CAD build for the part. Positions are in the model's coordinates, mm. A direction names the side the tool comes from. Coordinates: 2 decimals unless noted, no trailing zeros. Order: outer loops, then holes, each group sorted by start corner. A loop starts at its lowest first (then second) coordinate and runs counter-clockwise, first axis right, second up. Notation, with made-up numbers: (76, 47) - (87, 47) arc R14 cw to (87, 56) - close; hole circle Ø9 at (15.5, 49.25). An arc over 180 degrees is marked (long way). Return JSON: item names as keys, results as strings.
Autodesk Inventor part; units mm, degrees
ref_plane "YZ Plane" through (0, 0, 0) normal (1, 0, 0) x (0, 1, 0)
ref_plane "XZ Plane" through (0, 0, 0) normal (0, 1, 0) x (-1, 0, 0)
ref_plane "XY Plane" through (0, 0, 0) normal (0, 0, 1) x (1, 0, 0)
sketch "Sketch2" plane through (0, 0, 0) normal (1, 0, 0) x (0, 1, 0)
  line L0 (16.0342, 2.2983) -> (13.213, 1.278)
  line L1 (13.213, 1.278) -> (17.9745, -11.8874)
  line L2 (17.9745, -11.8874) -> (20.7956, -10.8671)
  line L3 (20.7956, -10.8671) -> (16.0342, 2.2983)
  line L4 (16.8006, 6.0599) -> (24.0368, -13.9485)
  line L5 (14.6738, 6.0599) -> (16.8006, 6.0599)
  line L6 (24.0368, -13.9485) -> (19.3349, -15.649)
  line L7 (19.3349, -15.649) -> (14.6738, -15.649)
  line L8 (22.156, -14.6287) -> (14.6738, 6.0599) construction
  line L9 (17.9745, -11.8874) -> (11.3917, -14.2681) construction
  line L10 (11.3917, -14.2681) -> (6.6303, -1.1027) construction
  line L11 (6.6303, -1.1027) -> (13.213, 1.278) construction
  line L12 (6.6738, 6.0599) -> (3.6738, 6.0599)
  line L13 (3.6738, 6.0599) -> (3.6738, -15.649)
  line L14 (3.6738, -15.649) -> (6.6738, -15.649)
  line L15 (14.6738, 6.0599) -> (14.6738, 9.0599)
  line L16 (14.6738, 9.0599) -> (6.6738, 9.0599)
  line L17 (6.6738, 9.0599) -> (6.6738, 6.0599)
  line L18 (6.6738, -15.649) -> (6.6738, -18.649)
  line L19 (6.6738, -18.649) -> (14.6738, -18.649)
  line L20 (14.6738, -18.649) -> (14.6738, -15.649)
  point P0 (0, 0)
  dimension "d9" = 5
  dimension "d11" = 2
  dimension "d13" = 4
  dimension "d14" = 4
  dimension "d15" = 14
  dimension "d16" = 7
  dimension "d17" = 3
  dimension "d18" = 3
  dimension "d21" = 3
  dimension "d22" = 3
  dimension "d27" = 21.7089
  dimension "d28" = 8
  dimension "d29" = 8
extrude "Extrusion1" add sketch "Sketch2" along normal blind 3
equation "\"d13\" = d14"
properties part number "k_thumb_profile"
Item 1: Band-saw the part on C-C, the plane y = 19.75. List the corners of the cut face in (x, z).
Findings below:
{"outline": "(0, -15.5) - (3, -15.5) - (3, -11.25) - (0, -11.25) - close; (0, -7.98) - (3, -7.98) - (3, -2.1) - (0, -2.1) - close"}
Item 2: Wall check: L1, parallel to Z at x = 2.4, y = 6.5; L2, parallel to Y at x = 0.6, z = -8; L3, parallel to Y at x = 2.2, z = -6.5. Give the ranges that are in metal, low to high. Write a range as [from, to].
Findings below:
{"L1": "z = [-15.65, 6.06]", "L2": "y = [3.67, 16.57], [19.76, 21.89]", "L3": "y = [3.67, 16.03], [19.22, 21.34]"}
Item 3: Which spindle directions (+Z, -Z, +X, -X, +Y, -Y) get a long thin tool onto all of the face, cutting with end or side? Do faces 1 (the flat face through (1, 14.674, 8)), 2 (the flat face through (1, 5, -15.649)), 3 (the flat face through (1.48, 18.45, -4.38)), 4 (the flat face through (1, 6.674, 8)). Say none if no direction does.
Findings below:
{"face 1": "+Z, +X, -X, +Y", "face 2": "-Z, +X, -X, -Y", "face 3": "+X, -X", "face 4": "+Z, +X, -X, -Y"}
Item 4: Band-saw the part on B-B, the plane x = 1.25. List the corners of the cut face in (y, z).
Findings below:
{"outline": "(3.67, -15.65) - (6.67, -15.65) - (6.67, -18.65) - (14.67, -18.65) - (14.67, -15.65) - (19.33, -15.65) - (24.04, -13.95) - (16.8, 6.06) - (14.67, 6.06) - (14.67, 9.06) - (6.67, 9.06) - (6.67, 6.06) - (3.67, 6.06) - close; hole (13.21, 1.28) - (17.97, -11.89) - (20.8, -10.87) - (16.03, 2.3) - close"}
Item 5: Band-saw the part on D-D, the plane z = 3.75. List the corners of the cut face in (x, y), then the cut area to 3 significant figures.
Findings below:
{"outline": "(0, 3.67) - (3, 3.67) - (3, 17.64) - (0, 17.64) - close", "area": "41.9 mm²"}
Item 6: Mould opens along Z. For faces 5 (the flat face through (1, 3.674, -5)), 6 (the flat face through (1.479, 14.643, 1.795)), 7 (the flat face through (1, 11, -18.649)) say: released by +Z, released by -Z, zero draft, split by the parting line, or undercut.
Findings below:
{"face 5": "zero draft", "face 6": "undercut", "face 7": "released by -Z"}
Item 7: Drop flat-ended pins along their axis: P1, Ø1, axis at x = 0.5, y = 15.5, coming from the -Z side; P2, Ø1.5, axis at x = 2, y = 5, coming from the +Z side; P3, Ø0.9, axis at x = 2, z = 7.5, coming from the +Y side. Give the stop position or say it passes through.
Findings below:
{"P1": "stops at z = -15.65", "P2": "stops at z = 6.06", "P3": "stops at y = 14.67"}
Item 8: Band-saw the part on A-A, the plane z = -2.75. List the corners of the cut face in (x, y), then the cut area to 3 significant figures.
Findings below:
{"outline": "(0, 3.67) - (3, 3.67) - (3, 14.67) - (0, 14.67) - close; (0, 17.86) - (3, 17.86) - (3, 19.99) - (0, 19.99) - close", "area": "39.4 mm²"}
